Answer from the drawing. Dimensions are ordinates in mm from the lowest x, y and z of the part. Coordinates: 2 decimals unless noted, no trailing zeros. Write each loop counter-clockwise with the first axis right and the second up, starting at its lowest first coordinate (ties: lowest second). Pieces come first, ordered by that corner, then holes. Notation, with made-up numbers: (87, 67.5) -> (103, 67.5) arc R23 ccw to (103, 86.5) -> close; hole circle Ø3 at (38, 11.25). An arc over 180 degrees is marked (long way). One line per item, written item: value. Start each with the question number.
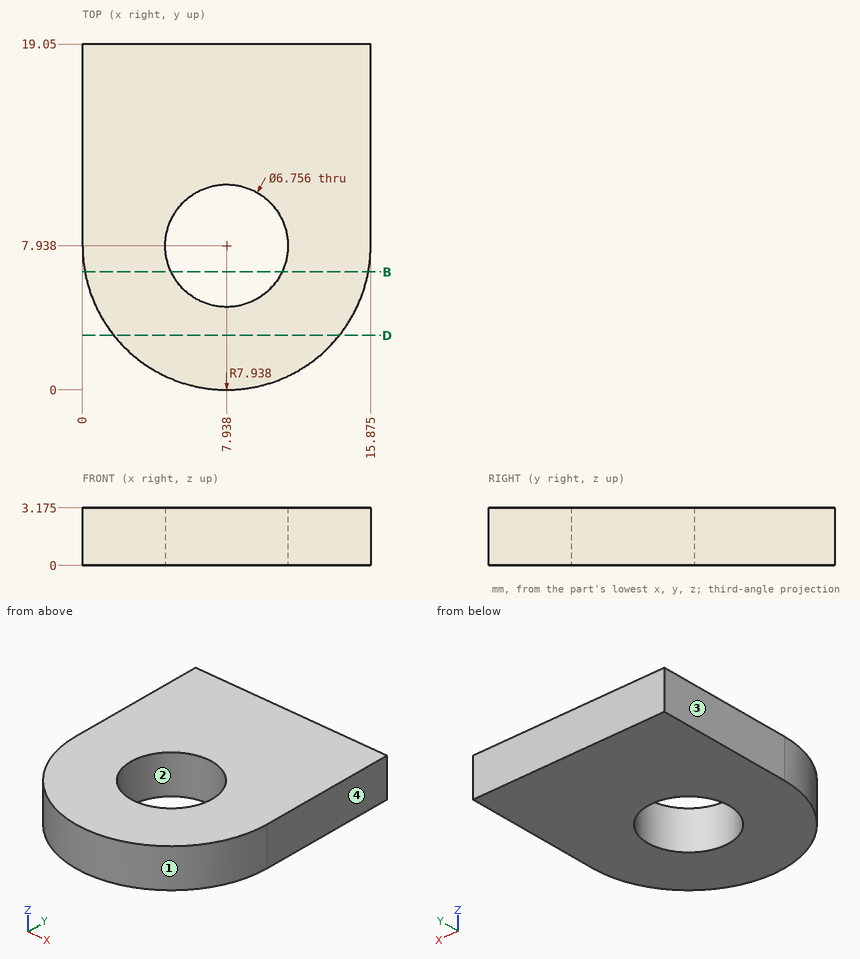
1. Find the intervals of material crossed by probe 1 along X at (y, z) = (8.25, 1.75) (1 decimal); probe 2 along X at (y, z) = (2.25, 0.8) (1 decimal); probe 3 along X at (y, z) = (8.75, 2.65) (1 decimal), in increasing order. Write a range as from..to.
2. A cutting plane is placed at D-D on y = 3. Give the vertices of the cut face in (x, z) (1 decimal).
3. A cutting plane is placed at B-B on y = 6.5. Give the vertices of the cut face in (x, z) (1 decimal).
4. For a pull along X with two mould halves and no side action, classify the marked faces 1, 2, 3 and 4 as +X half, -X half, draft (parallel to the pull), parting line (faces both ways), or undercut.
Derived:
1. probe 1: x = 0..4.6, 11.3..15.9
1. probe 2: x = 2.4..13.5
1. probe 3: x = 0..4.7, 11.2..15.9
2. outline: (1.7, 0) -> (14.2, 0) -> (14.2, 3.2) -> (1.7, 3.2) -> close
3. outline: (0.1, 0) -> (4.9, 0) -> (4.9, 3.2) -> (0.1, 3.2) -> close; (11, 0) -> (15.7, 0) -> (15.7, 3.2) -> (11, 3.2) -> close
4. face 1: parting line
4. face 2: undercut
4. face 3: -X half
4. face 4: +X half
